Verification items for the finished model (mm, model axes). A direction names the side the tool comes from. Give positions to 0.01 mm unless a question says otherwise; leave off trailing zeros. Order: outer loops, then holes, each group sorted by start corner. A loop starts at its lowest first (then second) coordinate and runs counter-clockwise, first axis right, second up. Notation, with made-up numbers: (-21, 1) -> (28, 1) arc R11 cw to (28, 7) -> close; hole circle Ø11 at (81.5, 49.5). An arc over 180 degrees is marked (long way). One line per question, with ' | ' between items. Start each with the question number.
Q1. Go/stop test with flat-tipped pins: pin 1 (1 mm diameter, centred on x = -1, y = -66, fed in from +Z); pin 2 (2 mm diameter, centred on x = 8, z = -6.5, fed in from -Y); pin 3 (3 mm diameter, centred on x = 6, z = -3, fed in from +Y); pin 4 (5 mm diameter, centred on x = 10.5, z = -7, fed in from -Y). Record where each tip stops, or that it passes through.
Q2. Section check C-C on y = -48.5. Record the cut outline in (x, z).
Q3. Mould release check, pull along Y, two halves, no side actions. Record for faces 1 (the flat face through (0, -44, 0)), 2 (the cylindrical face through (-8.68, -27.15, -4.68)), 3 (the flat face through (-11.78, -25.39, -4.68)), 4 (the cylindrical face through (7.98, -27.17, -4.68)): released by +Y, released by -Y, zero draft, split by the parting line, or undercut.
Q4. Access from +Z, -Z, +X, -X, +Y, -Y to the whole of each face (thin tool, end or side, straight path). Record for faces 5 (the flat face through (-13.72, -32.53, -4.68)), 6 (the flat face through (-5.165, -30, -5)).
Q5. Section check D-D on y = -42.5. Record the cut outline in (x, z).
Q6. Section check A-A on z = -6.75. Record the cut outline in (x, y), plus the area to 3 significant figures.
Q7. Section check B-B on x = 8.75. Record the cut outline in (y, z), plus the area to 3 significant figures.
Q8. Material ranges on probe 1 along Y at (x, z) = (5.75, -7.5); probe 2 along Y at (x, z) = (8.5, -2.75); probe 3 along X at (y, z) = (-31.5, -0.75), recorded low to high. Write a range as [from, to].
from build123d import *

# Parameters (mm, degrees)
BOSS_EXTRUDE1_DEPTH = 9.5


with BuildPart() as part:
    # Sketch1 → Boss-Extrude1 (new body)
    with BuildSketch(Plane.XY):
        with BuildLine():
            Line((-5.165155755, -27.675045296), (-5.165155755, -33.10368941))
            ThreePointArc((-5.165155755, -33.10368941), (-9.346333037, -32.518171884), (-13.463522621, -31.583386259))
            Line((-13.463522621, -31.583386259), (-13.987965753, -33.513401647))
            ThreePointArc((-13.987965753, -33.513401647), (-9.521266094, -34.519064332), (-4.983625309, -35.129457142))
            Line((-4.983625309, -35.129457142), (-2.624414585, -75.34))
            Line((-2.624414585, -75.34), (2.024414585, -75.34))
            Line((2.024414585, -75.34), (4.383625309, -35.129457142))
            ThreePointArc((4.383625309, -35.129457142), (8.921266094, -34.519064332), (13.387965753, -33.513401647))
            Line((13.387965753, -33.513401647), (12.863522621, -31.583386259))
            ThreePointArc((12.863522621, -31.583386259), (8.746333037, -32.518171884), (4.565155755, -33.10368941))
            Line((4.565155755, -33.10368941), (4.565155755, -27.675045296))
            ThreePointArc((4.565155755, -27.675045296), (8.031839973, -27.15841027), (11.447526164, -26.372344709))
            Line((11.447526164, -26.372344709), (10.923083031, -24.44232932))
            ThreePointArc((10.923083031, -24.44232932), (-0.3, -25.94), (-11.523083031, -24.44232932))
            Line((-11.523083031, -24.44232932), (-12.047526164, -26.372344709))
            ThreePointArc((-12.047526164, -26.372344709), (-8.631839973, -27.15841027), (-5.165155755, -27.675045296))
        make_face()
    extrude(amount=-BOSS_EXTRUDE1_DEPTH)


solid = part.part
Filled in:
1) pin 1: z = 0 | pin 2: y = -34.83 | pin 3: y = -25.22 | pin 4: y = -34.68
2) outline: (-4.2, -9.5) -> (3.6, -9.5) -> (3.6, 0) -> (-4.2, 0) -> close
3) face 1: zero draft | face 2: undercut | face 3: released by +Y | face 4: undercut
4) face 5: +Z, -Z, -X, +Y | face 6: +Z, -Z
5) outline: (-4.55, -9.5) -> (3.95, -9.5) -> (3.95, 0) -> (-4.55, 0) -> close
6) outline: (-13.99, -33.51) arc R52.2 ccw to (-4.98, -35.13) -> (-2.62, -75.34) -> (2.02, -75.34) -> (4.38, -35.13) arc R52.2 ccw to (13.39, -33.51) -> (12.86, -31.58) arc R50.2 cw to (4.57, -33.1) -> (4.57, -27.68) arc R44.8 ccw to (11.45, -26.37) -> (10.92, -24.44) arc R42.8 cw to (-11.52, -24.44) -> (-12.05, -26.37) arc R44.8 ccw to (-5.17, -27.68) -> (-5.17, -33.1) arc R50.2 cw to (-13.46, -31.58) -> close | area: 434 mm²
7) outline: (-34.55, -9.5) -> (-32.52, -9.5) -> (-32.52, 0) -> (-34.55, 0) -> close; (-27.02, -9.5) -> (-24.97, -9.5) -> (-24.97, 0) -> (-27.02, 0) -> close | area: 38.7 mm²
8) probe 1: [-34.99, -32.97], [-27.53, -25.51] | probe 2: [-34.59, -32.56], [-27.07, -25.03] | probe 3: [-5.17, 4.57]
